Here's how the part is built. I have some questions about the finished solid (model axes, mm). Face numbers are marked on the shaded views. A direction names the side the tool comes from. Give positions to 0.01 mm unless a question says otherwise; leave off trailing zeros. Write each loop counter-clockwise with the first axis right and the second up, starting at its lowest first coordinate (ties: lowest second). Pieces come first, ordered by that corner, then holes. Notation, with made-up numbers: (-21.5, 67.25) -> (5.5, 67.25) arc R30 ccw to (5.5, 92.25) -> close; hole circle Ø9 at (3.25, -1). An arc over 180 degrees is marked (long way). Return JSON: item names as keys, results as strings.
Autodesk Inventor part; units mm, degrees
ref_plane "YZ Plane" through (0, 0, 0) normal (1, 0, 0) x (0, 1, 0)
ref_plane "XZ Plane" through (0, 0, 0) normal (0, 1, 0) x (-1, 0, 0)
ref_plane "XY Plane" through (0, 0, 0) normal (0, 0, 1) x (1, 0, 0)
sketch "Sketch1" plane through (0, 0, 0) normal (0, 1, 0) x (-1, 0, 0)
  line L0 (-3.0388, 7.0833) -> (-6.0388, 7.0833)
  line L1 (-6.0388, 7.0833) -> (-6.0388, -12.9167)
  line L2 (-6.0388, -12.9167) -> (-3.0388, -12.9167)
  line L3 (-3.0388, -12.9167) -> (-3.0388, -2.9167)
  line L4 (-3.0388, -2.9167) -> (14.9612, -2.9167)
  line L5 (14.9612, -12.9167) -> (17.9612, -12.9167)
  line L6 (17.9612, -12.9167) -> (17.9612, 7.0833)
  line L7 (17.9612, 7.0833) -> (14.9612, 7.0833)
  line L8 (14.9612, 7.0833) -> (14.9612, 6.0833)
  line L9 (14.9612, 6.0833) -> (15.7112, 6.0833)
  line L10 (15.7112, 6.0833) -> (15.7112, 3.5833)
  line L11 (15.7112, 3.5833) -> (14.9612, 3.5833)
  line L12 (14.9612, 3.5833) -> (14.9612, -0.9167)
  line L13 (14.9612, -0.9167) -> (-3.0388, -0.9167)
  line L14 (-3.0388, -0.9167) -> (-3.0388, 3.5833)
  line L15 (-3.7888, 3.5833) -> (-3.7888, 6.0833)
  line L16 (-3.7888, 6.0833) -> (-3.0388, 6.0833)
  line L17 (-3.0388, 3.5833) -> (-3.7888, 3.5833)
  line L18 (-3.0388, 6.0833) -> (-3.0388, 7.0833)
  line L19 (14.9612, -12.9167) -> (14.9612, -2.9167)
  line L20 (-6.0388, 7.0833) -> (-6.0388, 34.0833)
  line L21 (-6.0388, 34.0833) -> (-9.0388, 34.0833)
  line L22 (-9.0388, 34.0833) -> (-9.0388, -37.9167)
  line L23 (-9.0388, -37.9167) -> (-6.0388, -37.9167)
  line L24 (-6.0388, -37.9167) -> (-6.0388, -12.9167)
  point P0 (0, 0)
  point P1 (14.9612, 1.3333)
  dimension "d0" = 2.5
  dimension "d1" = 3
  dimension "d2" = 3
  dimension "d3" = 10
  dimension "d4" = 10
  dimension "d5" = 2
  dimension "d6" = 3
  dimension "d8" = 1
  dimension "d9" = 8
  dimension "d11" = 0.75
  dimension "d12" = 0.75
  dimension "d13" = 3
  dimension "d16" = 18
  dimension "d17" = 3
  dimension "d18" = 72
  dimension "d19" = 35
extrude "Extrusion1" add sketch "Sketch1" along normal blind 10
fillet "Fillet1" radius 2 4 edges at (6.0388, 5, 7.0833) (6.0388, 5, -12.9167) (3.0388, 5, -12.9167) (3.0388, 5, 7.0833)
sketch "Sketch2" plane through (6.0388, 0, 34.0833) normal (-1, 0, 0) x (0, 0, 1)
  circle A0 centre (-5.875, 5) radius 3
  circle A1 centre (-66.125, 5) radius 3
  line L0 (-72, 0) -> (-49, 0)
  line L1 (-72, 10) -> (-49, 10)
  line L2 (-25, 10) -> (0, 10)
  line L3 (0, 0) -> (0, 10)
  line L4 (-72, 0) -> (-72, 10)
  point P0 (-34.0833, 0)
  dimension "d21" = 6
  dimension "d22" = 6
  dimension "d23" = 10
  dimension "d24" = 5
  dimension "d25" = 5
  dimension "d26" = 60.25
  dimension "d27" = 72
  dimension "d28" = 5.875
extrude "Extrusion2" cut sketch "Sketch2" against normal through all
equation "\"d2\" = d1"
equation "\"d4\" = d3"
equation "\"d6\" = d2"
equation "\"d12\" = d11"
equation "\"d13\" = d1"
equation "\"d19\" = -0.5 * d5 + 0.5 * d18"
equation "\"d24\" = 0.5 * d23"
equation "\"d25\" = 0.5 * d23"
equation "\"d28\" = -0.5 * d26 + 0.5 * d27"
properties part number "CO-1-01-stepperControllerMount"
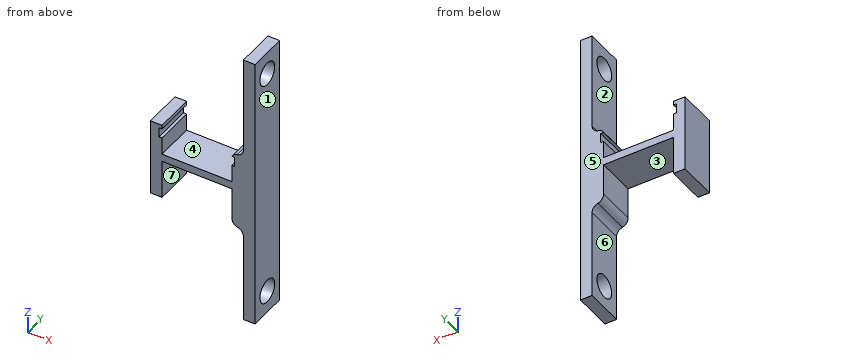
1. For pin 1 Ø3.5 at (x, y) = (-17, 5) entering from -Z; pin 2 Ø5 at (x, y) = (-7.5, 7) entering from +Z; pin 3 Ø8 at (x, z) = (-1, -15.5) entering from +Y; pin 4 Ø0.6 at (x, y) = (-15.5, 6.5) entering from +Z, each with a flat end and sliding along its axis, tell me the tip position at first contact or that it passes through.
Taken from the geometry:
{"pin 1": "stops at z = -12.92", "pin 2": "stops at z = -0.92", "pin 3": "passes through", "pin 4": "stops at z = 7.08"}
2. Suppose I cut it at D-D, the plane z = 20. List the corners of the cut face in (x, y) for me.
Taken from the geometry:
{"outline": "(6.04, 0) -> (9.04, 0) -> (9.04, 10) -> (6.04, 10) -> close"}
3. Suppose I cut it at C-C, the plane y = 9.25. List the corners of the cut face in (x, z) for me, and give its area (3 significant figures).
Taken from the geometry:
{"outline": "(-17.96, -12.92) -> (-14.96, -12.92) -> (-14.96, -2.92) -> (3.04, -2.92) -> (3.04, -11.04) arc R2 ccw to (4.54, -12.98) arc R2 cw to (6.04, -14.92) -> (6.04, -37.92) -> (9.04, -37.92) -> (9.04, 34.08) -> (6.04, 34.08) -> (6.04, 9.08) arc R2 cw to (4.43, 7.12) arc R2 ccw to (3.04, 6.08) -> (3.79, 6.08) -> (3.79, 3.58) -> (3.04, 3.58) -> (3.04, -0.92) -> (-14.96, -0.92) -> (-14.96, 3.58) -> (-15.71, 3.58) -> (-15.71, 6.08) -> (-14.96, 6.08) -> (-14.96, 7.08) -> (-17.96, 7.08) -> close", "area": "369 mm²"}
4. Suppose I cut it at A-A, the plane y = 5. Count the separate pieces of the cut face and the enclosed holes in it, and give its area (3 significant figures).
Taken from the geometry:
{"separate pieces": "3", "enclosed holes": "0", "area": "333 mm²"}
5. If we mould it in two halves opening along X, with no side actions, what happens to the marked faces 4, 5, 6 and 7? For each: released by +X, released by -X, zero draft, split by the parting line, or undercut.
Taken from the geometry:
{"face 4": "undercut", "face 5": "zero draft", "face 6": "released by -X", "face 7": "undercut"}
6. Which directions (+Z, -Z, +X, -X, +Y, -Y) give clear straight access to the entire face, cutting with the end or side of a thin tool? Please do the marked faces 1, 2 and 3.
Taken from the geometry:
{"face 1": "+Z, -Z, +X, +Y, -Y", "face 2": "+Z, -X, +Y, -Y", "face 3": "-Z, +Y, -Y"}
7. If I drill on line 1 (X direction, y = 4.5, z = -5); line 2 (Z direction, x = 0, y = 6.5); line 3 (X direction, y = 1.5, z = -29.5), over which ranges is the centre line in solid material (lowest first)? Write a range as [from, to].
Taken from the geometry:
{"line 1": "x = [-17.96, -14.96], [3.04, 9.04]", "line 2": "z = [-2.92, -0.92]", "line 3": "x = [6.04, 9.04]"}
8. Suppose I cut it at B-B, the plane x = -10.25. List the corners of the cut face in (y, z) for me, and give its area (3 significant figures).
Taken from the geometry:
{"outline": "(0, -2.92) -> (10, -2.92) -> (10, -0.92) -> (0, -0.92) -> close", "area": "20.0 mm²"}
